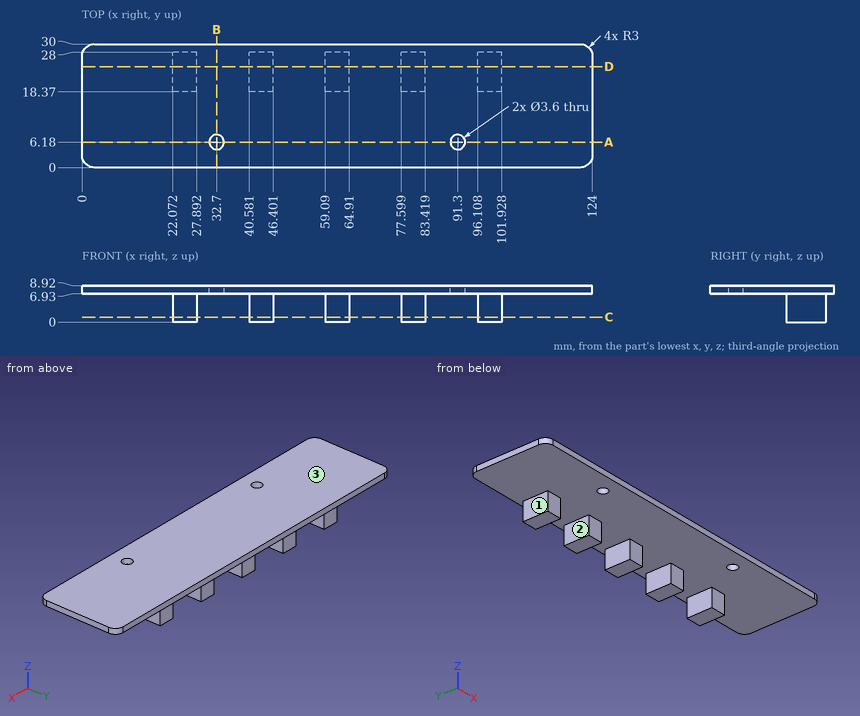
Verification items for this drawing (mm, ordinates from the low corner). Coordinates: 2 decimals unless noted, no trailing zeros. Write each loop counter-clockwise with the first axis right and the second up, starting at its lowest first coordinate (ties: lowest second). Pieces come first, ordered by that corner, then holes. Notation, with made-up numbers: M 70,4.25 L 126,4.25 A20 ccw 126,11.25 Z; hole C -23,66.5 d2. An arc over 180 degrees is marked long. Answer as a JSON object with one key per item and string values. Group by question number.
(1) Cross-section at C-C, the plane z = 1.25. Record the cut outline in (x, y), and give its area (3 significant figures).
(2) Cross-section at D-D, the plane y = 24.5. Record the cut outline in (x, z), and give its area (3 significant figures).
(3) Cross-section at B-B, the plane x = 32.7. Record the cut outline in (y, z), and give its area (3 significant figures).
(4) Cross-section at A-A, the plane y = 6.18. Record the cut outline in (x, z), and give its area (3 significant figures).
(5) Material ranges on line 1 (X direction, y = 26.5, z = 4); line 2 (Y direction, x = 32.7, z = 8.1); line 3 (X direction, y = 5, z = 7.5), recorded low to high.
(6) Gauge pin test, flat ends, axial feed: pin 1 (4.5 mm diameter, centred on x = 25.5, z = 3.5, fed in from -Y); pin 2 (1.7 mm diameter, centred on x = 63.5, z = 4, fed in from +Y); pin 3 (3.5 mm diameter, centred on y = 22, z = 2.5, fed in from +X). Record the tip position at first contact, or that the pin passes through.
(7) Release check for a two-part mould opening along X. For the marked faces 1, 2 and 3 record: +X half, -X half, draft (parallel to the pull), parting line (faces both ways), or undercut.
Reply:
{
 "1": {"outline": "M 22.07,18.37 L 27.89,18.37 L 27.89,28 L 22.07,28 Z; M 40.58,18.37 L 46.4,18.37 L 46.4,28 L 40.58,28 Z; M 59.09,18.37 L 64.91,18.37 L 64.91,28 L 59.09,28 Z; M 77.6,18.37 L 83.42,18.37 L 83.42,28 L 77.6,28 Z; M 96.11,18.37 L 101.93,18.37 L 101.93,28 L 96.11,28 Z", "area": "280 mm²"},
 "2": {"outline": "M 0,6.93 L 22.07,6.93 L 22.07,0 L 27.89,0 L 27.89,6.93 L 40.58,6.93 L 40.58,0 L 46.4,0 L 46.4,6.93 L 59.09,6.93 L 59.09,0 L 64.91,0 L 64.91,6.93 L 77.6,6.93 L 77.6,0 L 83.42,0 L 83.42,6.93 L 96.11,6.93 L 96.11,0 L 101.93,0 L 101.93,6.93 L 124,6.93 L 124,8.92 L 0,8.92 Z", "area": "448 mm²"},
 "3": {"outline": "M 0,6.93 L 4.38,6.93 L 4.38,8.92 L 0,8.92 Z; M 7.98,6.93 L 30,6.93 L 30,8.92 L 7.98,8.92 Z", "area": "52.5 mm²"},
 "4": {"outline": "M 0,6.93 L 30.9,6.93 L 30.9,8.92 L 0,8.92 Z; M 34.5,6.93 L 89.5,6.93 L 89.5,8.92 L 34.5,8.92 Z; M 93.1,6.93 L 124,6.93 L 124,8.92 L 93.1,8.92 Z", "area": "232 mm²"},
 "5": {"line 1": "22.07 to 27.89, 40.58 to 46.4, 59.09 to 64.91, 77.6 to 83.42, 96.11 to 101.93", "line 2": "0 to 4.38, 7.98 to 30", "line 3": "0 to 31.34, 34.06 to 89.94, 92.66 to 124"},
 "6": {"pin 1": "y = 18.37", "pin 2": "y = 28", "pin 3": "x = 101.93"},
 "7": {"face 1": "-X half", "face 2": "undercut", "face 3": "draft"}
}
